Here's how the part is built. I have some questions about the finished solid (model axes, mm). Face numbers are marked on the shaded views. A direction names the side the tool comes from. Coordinates: 2 decimals unless noted, no trailing zeros. Write each loop counter-clockwise with the first axis right and the second up, starting at its lowest first coordinate (ties: lowest second). Pieces come first, ordered by that corner, then holes. Notation, with made-up numbers: (37, 56) -> (42, 56) arc R38 cw to (42, 94) -> close; hole circle Ø11 at (85, -27). An arc over 180 degrees is marked (long way). Use a Markdown table: item, result. Add a question column.
```python
from build123d import *

# Parameters (mm, degrees)
F0_W     = 76.2
F0_H     = 101.6
F1_DEPTH = 3.048
F2_W     = 25.238578
F2_H     = 3.048
F2_W_2   = 3.048
F2_H_2   = 21.454054
F2_W_3   = 14.951317
F2_H_3   = 22.784396
F2_W_4   = 24.933161
F2_H_4   = 21.244367
F2_H_5   = 21.031751
F2_W_5   = 19.353797
F2_H_6   = 20.421157
F2_W_6   = 25.804729
F3_DEPTH = 12.7
F4_W     = 25.238578
F4_H     = 3.048
F5_DEPTH = 3.048


with BuildPart() as f1:
    # F0 (on Top) → F1 (new body)
    with BuildSketch(Plane.XY):
        Rectangle(F0_W, F0_H)
    extrude(amount=F1_DEPTH)

    # F2 (on face) → F3 (join)
    with BuildSketch(Plane.XY.offset(3.048)):
        with Locations((-25.480711, 49.276)):
            Rectangle(F2_W, F2_H)
        with Locations((25.480711, 49.276)):
            Rectangle(F2_W, F2_H)
        with Locations((0.076681, 40.072973)):
            Rectangle(F2_W_2, F2_H_2)
        with Locations((-20.530921, 25.026575)):
            Rectangle(F2_W_3, F2_H)
        with Locations((-36.576, 25.297143)):
            Rectangle(F2_W_2, F2_H_3)
        with Locations((20.530921, 25.026575)):
            Rectangle(F2_W_3, F2_H)
        with Locations((36.576, 25.297143)):
            Rectangle(F2_W_2, F2_H_3)
        with Locations((25.63342, -0.061376)):
            Rectangle(F2_W_4, F2_H)
        with Locations((0.098287, -1.087287)):
            Rectangle(F2_W_2, F2_H_4)
        with Locations((-25.63342, -0.061376)):
            Rectangle(F2_W_4, F2_H)
        with Locations((-36.576, -24.127469)):
            Rectangle(F2_W_2, F2_H_5)
        with Locations((-15.968946, -21.239439)):
            Rectangle(F2_W_5, F2_H)
        with Locations((15.968946, -21.239439)):
            Rectangle(F2_W_5, F2_H)
        with Locations((36.576, -24.127469)):
            Rectangle(F2_W_2, F2_H_5)
        with Locations((-0.069343, -40.589422)):
            Rectangle(F2_W_2, F2_H_6)
        with Locations((-25.197636, -49.276)):
            Rectangle(F2_W_6, F2_H)
        with Locations((25.197636, -49.276)):
            Rectangle(F2_W_6, F2_H)
    extrude(amount=F3_DEPTH)

    # F4 (on face) → F5 (join)
    with BuildSketch(Plane.XY.offset(15.748)):
        Polygon((38.100678, 50.8), (-12.861422, 50.8), (-12.861422, 47.752), (-38.1, 47.752), (-38.1, -50.800964), (38.100678, -50.800964), align=None)
        with Locations((-25.480711, 49.276)):
            Rectangle(F4_W, F4_H)
    extrude(amount=F5_DEPTH)


solid = f1.part
```
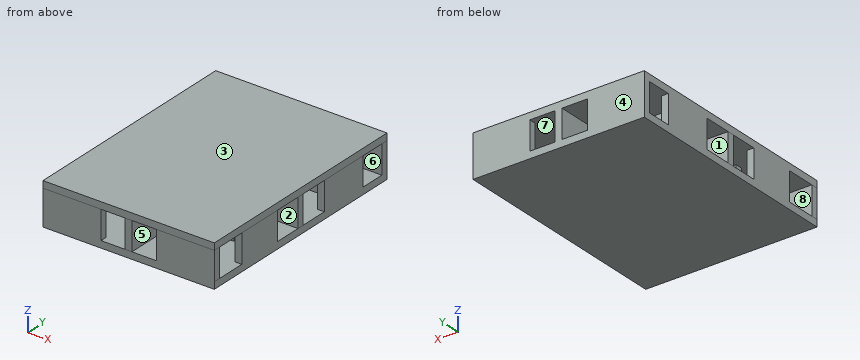
Q1. Please list where these lines run through material, in increasing order: line 1 (Y direction, x = 29.5, z = 10.5); line 2 (Y direction, x = -22.5, z = 8.25); line 3 (X direction, y = 34, z = 14.75).
Q2. Suppose I cut it at B-B, the plane x = -30. State how many separate pieces and enclosed holes the cut face has, and give its area (3 significant figures).
Q3. Will these pins go through, and if not, where does the flat tip stop? pin 1 (4 mm diameter, centred on y = -40, z = 8, fed in from +X); pin 2 (1 mm diameter, centred on y = -36.5, z = 11, fed in from -X); pin 3 (5 mm diameter, centred on x = 5.5, z = 10, fed in from -Y).
Q4. Thinking about a two-plate mould opening in Y: for the marked faces 1, 2, 3 and 4, which applies, released by +Y, released by -Y, zero draft, split by the parting line, or undercut?
Q5. Suppose I cut it at C-C, the plane y = -38. Write out the boundary of the cut face in (x, z), and give its area (3 significant figures).
Q6. Suppose I cut it at A-A, the plane x = -3.5. Write out the boundary of the cut face in (y, z).
Q7. Which directions (+Z, -Z, +X, -X, +Y, -Y) give clear straight access to the entire face, cutting with the end or side of a thin tool? Please do the marked faces 5, 6, 7 and 8.
Answer key:
| question | item | result |
|---|---|---|
| 1 | line 1 | y = -50.8 to -47.75, -1.59 to 1.46, 47.75 to 50.8 |
| 1 | line 2 | y = -50.8 to -47.75, -22.76 to -19.72, -1.59 to 1.46, 23.5 to 26.55, 47.75 to 50.8 |
| 1 | line 3 | x = -38.1 to -35.05, -1.45 to 1.6, 35.05 to 38.1 |
| 2 | separate pieces | 1 |
| 2 | enclosed holes | 2 |
| 2 | area | 735 mm^2 |
| 3 | pin 1 | stops at x = 1.45 |
| 3 | pin 2 | stops at x = -1.59 |
| 3 | pin 3 | stops at y = -22.76 |
| 4 | face 1 | undercut |
| 4 | face 2 | undercut |
| 4 | face 3 | zero draft |
| 4 | face 4 | released by +Y |
| 5 | outline | (-38.1, 0) -> (38.1, 0) -> (38.1, 3.05) -> (1.45, 3.05) -> (1.45, 15.75) -> (38.1, 15.75) -> (38.1, 18.8) -> (-38.1, 18.8) -> (-38.1, 15.75) -> (-1.59, 15.75) -> (-1.59, 3.05) -> (-38.1, 3.05) -> close |
| 5 | area | 503 mm^2 |
| 6 | outline | (-50.8, 0) -> (50.8, 0) -> (50.8, 3.05) -> (-50.8, 3.05) -> close; (-50.8, 15.75) -> (50.8, 15.75) -> (50.8, 18.8) -> (-50.8, 18.8) -> close |
| 7 | face 5 | -Y |
| 7 | face 6 | +X |
| 7 | face 7 | none |
| 7 | face 8 | -X |
